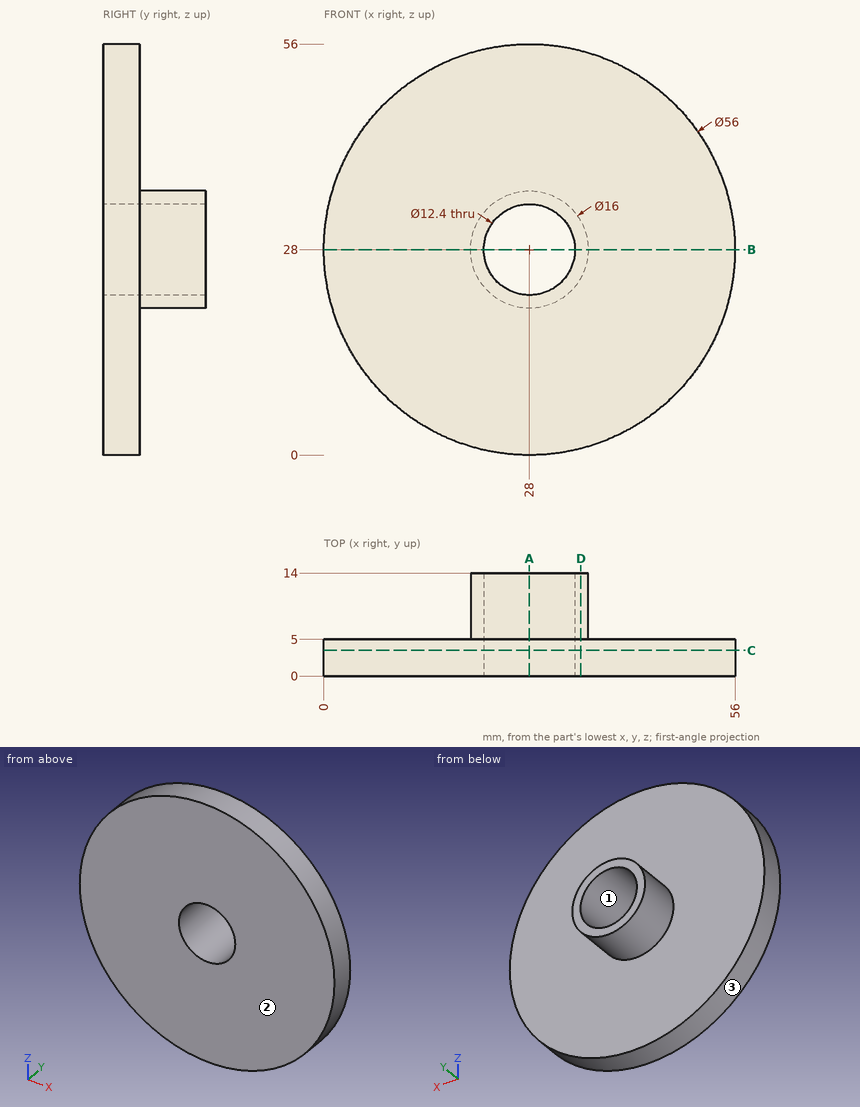
Could you check a few things on this drawing? It's one solid part, dimensions in mm from its lowest x, y, z. Coordinates: 2 decimals unless noted, no trailing zeros. Write each loop counter-clockwise with the first axis right and the second up, starting at its lowest first coordinate (ties: lowest second). Pieces come first, ordered by that corner, then holes. Notation, with made-up numbers: (44, 46.25) - (77, 46.25) arc R18 ccw to (77, 56.25) - close; hole circle Ø2 at (25.5, 87). An arc over 180 degrees is marked (long way). Put each result on its own line as item: value. Start each with the question number.
Q1. I want a section at D-D on x = 35. Write out the boundary of the cut face in (y, z).
Q2. I'm going to push flat-ended pins straight in: P1, Ø1, axis at x = 27, z = 33, coming from the -Y side; P2, Ø6, axis at x = 35, y = 4, coming from the -Z side; P3, Ø8, axis at x = 19.5, y = 8, coming from the +Z side; P4, Ø1, axis at x = 16, y = 4.5, coming from the -Z side. Where does each tip first touch, or does it pass through?
Q3. I want a section at C-C on y = 3.5. Write out the boundary of the cut face in (x, z), plus the area to 3 significant figures.
Q4. Please list where these lines run through material, in increasing order: L1, parallel to X at y = 11, z = 28; L2, parallel to X at y = 4.25, z = 31.5.
Q5. Thinking about a two-plate mould opening in Z: for the marked faces 1, 2 and 3, which applies, pulls with the +Z half, pulls with the -Z half, needs draft (parallel to the pull), parting line crosses it, or undercut?
Q6. I want a section at A-A on x = 28. Write out the boundary of the cut face in (y, z).
Q7. I want a section at B-B on z = 28. Write out the boundary of the cut face in (x, y), plus the area to 3 significant figures.
Checks:
1. outline: (0, 0.89) - (5, 0.89) - (5, 24.13) - (14, 24.13) - (14, 31.87) - (5, 31.87) - (5, 55.11) - (0, 55.11) - close
2. P1: through
2. P2: z = 0.29
2. P3: z = 55.38
2. P4: z = 2.47
3. outline: circle Ø56 at (28, 28); hole circle Ø12.4 at (28, 28)
3. area: 2,340 mm²
4. L1: 20 to 21.8, 34.2 to 36
4. L2: 0.22 to 22.88, 33.12 to 55.78
5. face 1: undercut
5. face 2: needs draft
5. face 3: parting line crosses it
6. outline: (0, 0) - (5, 0) - (5, 20) - (14, 20) - (14, 21.8) - (0, 21.8) - close; (0, 34.2) - (14, 34.2) - (14, 36) - (5, 36) - (5, 56) - (0, 56) - close
7. outline: (0, 0) - (21.8, 0) - (21.8, 14) - (20, 14) - (20, 5) - (0, 5) - close; (34.2, 0) - (56, 0) - (56, 5) - (36, 5) - (36, 14) - (34.2, 14) - close
7. area: 250 mm²
